Geometry check sheet. Reference: drawing and pictorial views, mm from the part's lowest x, y, z. A direction names the side the tool comes from. Round coordinates to 2 decimals unless told otherwise and drop trailing zeros. Write each loop counter-clockwise with the first axis right and the second up, starting at its lowest first coordinate (ties: lowest second). Pieces come first, ordered by that corner, then holes. Notation, with made-up numbers: M 24.5,76.5 L 82.5,76.5 A7 ccw 82.5,82.5 Z; hole C 19,-33.75 d9. An arc over 180 degrees is marked long. Answer in a Markdown table with one row per item. Add a question column.
1. Sectioned sample at D-D on x = 18.75. Record the cut outline in (y, z), plus the area to 3 significant figures.
2. Sectioned sample at C-C on y = 23. Record the cut outline in (x, z), plus the area to 3 significant figures.
3. Sectioned sample at B-B on x = 15.5. Record the cut outline in (y, z), plus the area to 3 significant figures.
4. Material ranges on probe 1 along Y at (x, z) = (15.75, 0.45); probe 2 along X at (y, z) = (22.5, 0.9); probe 3 along Y at (x, z) = (5.25, 1.9), recorded low to high.
5. Sectioned sample at A-A on z = 1.55. Record the cut outline in (x, y), plus the area to 3 significant figures.
6. Go/stop test with flat-tipped pins: pin 1 Ø1.5 at (y, z) = (20.5, 1) entering from -X; pin 2 Ø1.5 at (x, z) = (18.5, 1.5) entering from +Y; pin 3 Ø1 at (x, z) = (18.5, 1) entering from +Y (1 decimal); pin 4 Ø1.8 at (x, y) = (15.68, 38.61) entering from -Z. Record where each tip stops, or that it passes through.
7. Set-up check for the marked faces 1 and 2: record each of +Z, -Z, +X, -X, +Y, -Y from which the full face is reachable in a straight line by a thin tool's end or side.
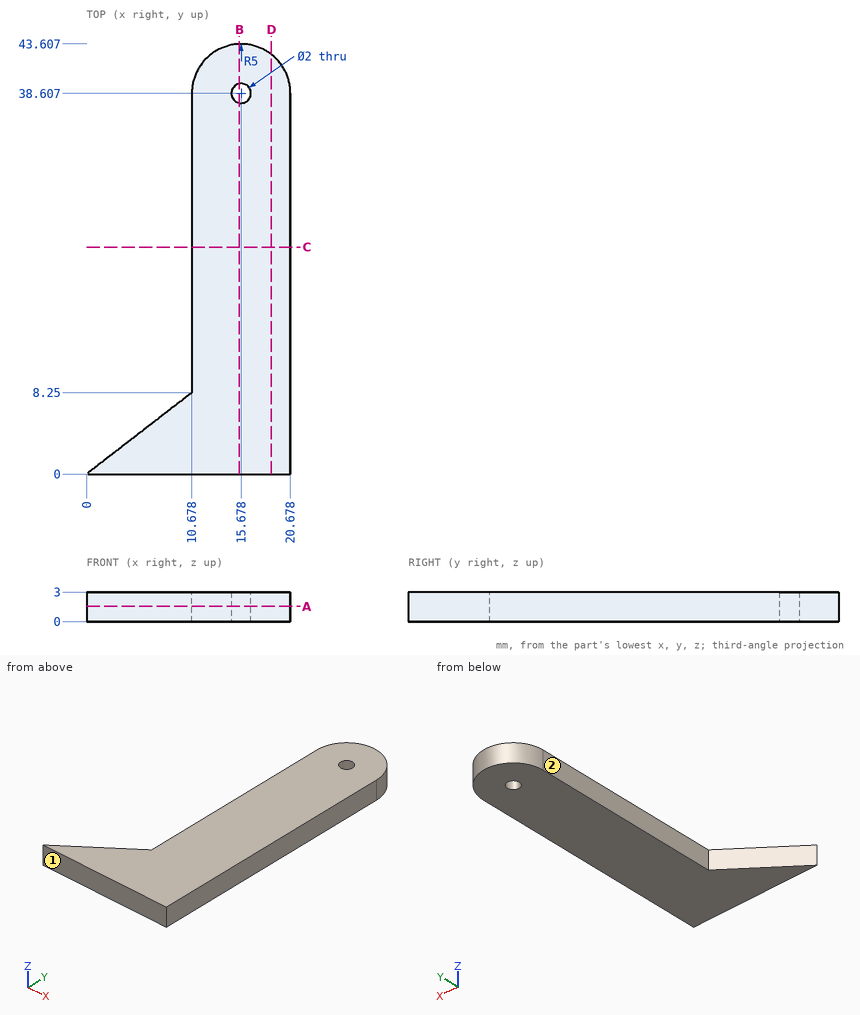
Geometry check:
| question | item | result |
|---|---|---|
| 1 | outline | M 0,0 L 42.55,0 L 42.55,3 L 0,3 Z |
| 1 | area | 128 mm2 |
| 2 | outline | M 10.68,0 L 20.68,0 L 20.68,3 L 10.68,3 Z |
| 2 | area | 30.0 mm2 |
| 3 | outline | M 0,0 L 37.62,0 L 37.62,3 L 0,3 Z; M 39.59,0 L 43.6,0 L 43.6,3 L 39.59,3 Z |
| 3 | area | 125 mm2 |
| 4 | probe 1 | y = 0 to 37.61, 39.6 to 43.61 |
| 4 | probe 2 | x = 10.68 to 20.68 |
| 4 | probe 3 | y = 0 to 4.06 |
| 5 | outline | M 0,0 L 20.68,0 L 20.68,38.61 A5 ccw 10.68,38.61 L 10.68,8.25 Z; hole C 15.68,38.61 d2 |
| 5 | area | 466 mm2 |
| 6 | pin 1 | stops at x = 10.68 |
| 6 | pin 2 | stops at y = 43.16 |
| 6 | pin 3 | stops at y = 43 |
| 6 | pin 4 | passes through |
| 7 | face 1 | +Z, -Z, +X, -X, -Y |
| 7 | face 2 | +Z, -Z, -X, +Y |
